```python
from build123d import *

# Parameters (mm, degrees)
EXTRUDE_1_DEPTH      = 11.5
EXTRUDE_1_DEPTH_BACK = 11.5
SKETCH_2_R           = 5
CUT_EXTRUDE_1_DEPTH  = 5
CHAMFER_1_SIZE       = 1
CHAMFER_2_SIZE       = 2


with BuildPart() as part:
    # Sketch 1 → Extrude 1 (new, two sides: drawn at the far end of the back side and taken through both)
    with BuildSketch(Plane.XY.offset(-EXTRUDE_1_DEPTH_BACK)):
        with BuildLine():
            Line((-105, 0), (-75, 0))
            ThreePointArc((-75, 0), (0, 29.784938454), (75, 0))
            Line((75, 0), (105, 0))
            Line((105, 0), (105, 9.5))
            Line((105, 9.5), (75, 9.5))
            Line((75, 9.5), (75, 5.414263011))
            ThreePointArc((75, 5.414263011), (0, 33.784938454), (-75, 5.414263011))
            Line((-75, 5.414263011), (-75, 9.5))
            Line((-75, 9.5), (-105, 9.5))
            Line((-105, 9.5), (-105, 0))
        make_face()
    extrude(amount=EXTRUDE_1_DEPTH + EXTRUDE_1_DEPTH_BACK)

    # Sketch 2 → Cut-Extrude 1 (cut)
    with BuildSketch(Plane(origin=(0, 9.5, 0), x_dir=(1, 0, 0), z_dir=(0, 1, 0))):
        with Locations(Location((-89.5, 0, 0), (0, 0, 270))):
            Circle(SKETCH_2_R)
        with Locations(Location((89.5, 0, 0), (0, 0, 90))):
            Circle(SKETCH_2_R)
    extrude(amount=-CUT_EXTRUDE_1_DEPTH, mode=Mode.SUBTRACT)

    # Chamfer 1
    chamfer_1_edges = [part.edges().sort_by_distance(p)[0] for p in [
        (0, 29.784938454, -11.5),
        (0, 33.784938454, -11.5),
        (0, 29.784938454, 11.5),
        (0, 33.784938454, 11.5),
    ]]
    chamfer(chamfer_1_edges, length=CHAMFER_1_SIZE)

    # Chamfer 2
    chamfer_2_edges = [part.edges().sort_by_distance(p)[0] for p in [
        (-105, 9.5, 0),
        (-75, 9.5, 0),
        (75, 9.5, 0),
        (105, 9.5, 0),
    ]]
    chamfer(chamfer_2_edges, length=CHAMFER_2_SIZE)


solid = part.part
```
Read the model definition and answer for the solid it produces. Units are mm, in the model's axes. A direction names the side the tool comes from. Give positions to 0.01 mm unless a question says otherwise; leave off trailing zeros. Write each loop counter-clockwise with the first axis right and the second up, starting at its lowest first coordinate (ties: lowest second). Pieces come first, ordered by that corner, then holes. Notation, with made-up numbers: (50, 89) -> (104, 89) arc R22 ccw to (104, 103) -> close; hole circle Ø1 at (73.25, -21). An arc over 180 degrees is marked (long way). Answer as a JSON object with one key per item and string values.
1) Section B-B on x = 89.5 is taken. Write down the section's boundary in (y, z), then the cut area to 4 significant figures.
Findings below:
{"outline": "(0, -11.5) -> (9.5, -11.5) -> (9.5, -5) -> (4.5, -5) -> (4.5, 5) -> (9.5, 5) -> (9.5, 11.5) -> (0, 11.5) -> close", "area": "168.5 mm^2"}
2) A tool of negligible diameter and unlimited length cuts with its end or side. For faces 1 (the flat face through (90, 0, 0)), 2 (the flat face through (90.2, 9.5, -5.3)), 3 (the flat face through (-89.8, 9.5, -5.3)), 4 (the conical face through (-1.17, 29.95, -10.67)), from which of +Z, -Z, +X, -X, +Y, -Y can it reach the whole face along a straight path? Write none if from no direction.
Findings below:
{"face 1": "+Z, -Z, +X, -X, -Y", "face 2": "+Z, -Z, +X, +Y", "face 3": "+Z, -Z, -X, +Y", "face 4": "-Z, -Y"}
3) Flat-ended cylindrical pins translate along their axes: pin 1 Ø6 at (y, z) = (13, -4) entering from +X; pin 2 Ø8 at (x, z) = (88.5, -0.5) entering from +Y; pin 3 Ø3 at (x, y) = (12.5, 27) entering from -Z; pin 4 Ø5 at (x, z) = (-89.5, -1.5) entering from +Y. Find the tip coordinate at first contact, or state that the pin passes through.
Findings below:
{"pin 1": "stops at x = 69.46", "pin 2": "stops at y = 9.5", "pin 3": "passes through", "pin 4": "stops at y = 4.5"}
4) Section A-A on z = -7.25 is taken. Write down the section's boundary in (x, y), then the cut area to 3 significant figures.
Findings below:
{"outline": "(-105, 0) -> (-75, 0) arc R109.32 cw to (75, 0) -> (105, 0) -> (105, 7.5) -> (103, 9.5) -> (77, 9.5) -> (75, 7.5) -> (75, 5.41) arc R113.32 ccw to (-75, 5.41) -> (-75, 7.5) -> (-77, 9.5) -> (-103, 9.5) -> (-105, 7.5) -> close", "area": "1,220 mm^2"}
5) Straight lines are drawn through the part: probe 1 along X at (y, z) = (6.65, 0); probe 2 along Z at (x, y) = (89.5, 5.9); probe 3 along X at (y, z) = (13.5, 4.5). For each, find the intervals that lie inside material, in ascending order. Write a range as from..to.
Findings below:
{"probe 1": "x = -105..-94.5, -84.5..-75, -73.58..-67.25, 67.25..73.58, 75..84.5, 94.5..105", "probe 2": "z = -11.5..-5, 5..11.5", "probe 3": "x = -64.7..-57.4, 57.4..64.7"}
6) For a pull along X with two mould halves and no side action, classify faces 5 (the flat face through (0, 31, -11.5)), 6 (the flat face through (105, 4, 0)), 7 (the cylindrical face through (-1.16, 29.78, -0.15)) as pulls with the +X half, pulls with the -X half, needs draft (parallel to the pull), parting line crosses it, or undercut.
Findings below:
{"face 5": "needs draft", "face 6": "pulls with the +X half", "face 7": "undercut"}
